Design review of the part built by this model. Coordinates are the model's own, in mm. Face numbers are marked on the shaded views. A direction names the side the tool comes from. Round coordinates to 2 decimals unless told otherwise and drop trailing zeros. Loops run counter-clockwise (first coordinate to the right, second up) from the corner with the lowest first, then second, coordinate; pieces in that order, holes last. Notation, with made-up numbers: (-10.5, 7) - (19.5, 7) arc R23 cw to (19.5, 17) - close; hole circle Ø5 at (40.25, 84). An arc over 180 degrees is marked (long way). Return JSON: item names as keys, results as strings. Group by question number.
(1) For the marked faces 1 and 2, list the 3-axis set-ups (+Z, -Z, +X, -X, +Y, -Y) from which the entire face can be reached by the end or side of a thin tool; tool diameter is ignored.
(2) We need section A-A, the plane x = 0. Write out the cut boundary in (y, z), and give its area (3 significant figures).
(3) We need section C-C, the plane y = 74. Write out the cut boundary in (x, z), and give its area (3 significant figures).
(4) Wall thickness on L1, parallel to Y at x = 8.35, z = 0; L2, parallel to X at y = 33.5, z = 0; L3, parallel to Z at x = -0.5, y = 9: over which ranges is each line inside the solid? List them lowest first. Write a range as [from, to].
(5) We need section B-B, the plane y = 62. Write out the cut boundary in (x, z), and give its area (3 significant figures).
(6) The part is to be moulded in two halves that separate along X. For the marked faces 3, 4 and 5, say which applies: pulls with the +X half, pulls with the -X half, needs draft (parallel to the pull), parting line crosses it, or undercut.
(7) Clearance check with flat-ended pins moving along their axes: pin 1 (1.5 mm diameter, centred on x = -5, y = 48.5, fed in from -Z); pin 2 (3 mm diameter, centred on y = 74, z = 0, fed in from +X); pin 3 (0.8 mm diameter, centred on y = -2, z = 0, fed in from +X); pin 4 (8 mm diameter, centred on y = 46.5, z = 6.5, fed in from +X). State where each tip first meets the part, or that it passes through.
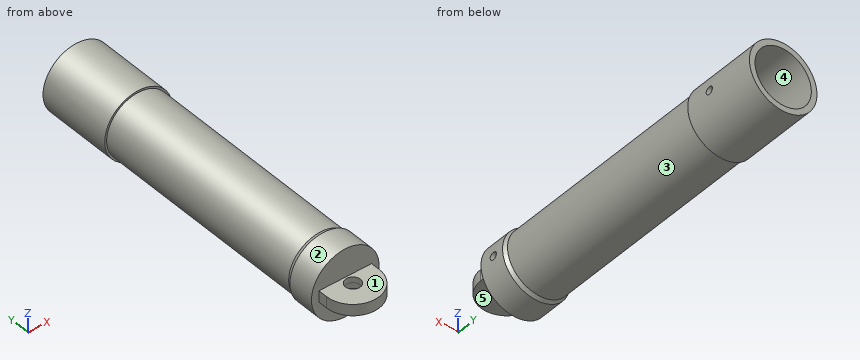
from build123d import *

# Parameters (mm, degrees)
SKETCH2_R                = 2
BOSS_EXTRUDE1_DEPTH      = 1.5
BOSS_EXTRUDE1_DEPTH_BACK = 1.5
SKETCH3_R                = 1
CUT_EXTRUDE1_DEPTH       = 50


with BuildPart() as part:
    # Sketch1 → Revolve1 (revolve)
    with BuildSketch(Plane.XY):
        Polygon((0, 0), (-9, 0), (-9, 7), (-8.5, 8), (-8.5, 67), (-9, 67), (-9, 87), (-7.5, 87), (-7.5, 2), (0, 2), align=None)
    revolve(axis=Axis((0, 87, 0), (0, -1, 0)))

    # Sketch2 → Boss-Extrude1 (add, two sides)
    with BuildSketch(Plane.XY) as boss_extrude1_sk:
        with BuildLine():
            Line((-7, 0), (7, 0))
            Line((7, 0), (7, -2.5))
            ThreePointArc((7, -2.5), (0, -9.5), (-7, -2.5))
            Line((-7, -2.5), (-7, 0))
        make_face()
        with Locations((0, -2.5)):
            Circle(SKETCH2_R, mode=Mode.SUBTRACT)
    extrude(amount=BOSS_EXTRUDE1_DEPTH)
    extrude(boss_extrude1_sk.sketch, amount=-BOSS_EXTRUDE1_DEPTH_BACK)

    # Sketch3 → Cut-Extrude1 (cut)
    with BuildSketch(Plane(origin=(0, 0, 0), x_dir=(0, 0, -1), z_dir=(1, 0, 0))):
        with Locations((0, 74)):
            Circle(SKETCH3_R)
        with Locations((0, 4)):
            Circle(SKETCH3_R)
    extrude(amount=CUT_EXTRUDE1_DEPTH, mode=Mode.SUBTRACT)


solid = part.part
Solutions:
{
 "1": {"face 1": "+Z, +X, -X, -Y", "face 2": "+Y, -Y"},
 "2": {"outline": "(-9.5, -1.5) - (-4.5, -1.5) - (-4.5, 1.5) - (-9.5, 1.5) - close; (-0.5, -1.5) - (0, -1.5) - (0, -9) - (7, -9) - (8, -8.5) - (67, -8.5) - (67, -9) - (87, -9) - (87, -7.5) - (2, -7.5) - (2, 7.5) - (87, 7.5) - (87, 9) - (67, 9) - (67, 8.5) - (8, 8.5) - (7, 9) - (0, 9) - (0, 1.5) - (-0.5, 1.5) - close", "area": "248 mm^2"},
 "3": {"outline": "(7.43, -1) arc R7.5 cw (long way) to (7.43, 1) - (8.94, 1) arc R9 ccw (long way) to (8.94, -1) - close", "area": "74.7 mm^2"},
 "4": {"L1": "[0, 3], [5, 73], [75, 87]", "L2": "[-8.5, -7.5], [7.5, 8.5]", "L3": "[-8.49, -7.48], [7.48, 8.49]"},
 "5": {"outline": "circle Ø17 at (0, 0); hole circle Ø15 at (0, 0)", "area": "50.3 mm^2"},
 "6": {"face 3": "parting line crosses it", "face 4": "undercut", "face 5": "needs draft"},
 "7": {"pin 1": "z = -7.36", "pin 2": "x = 9", "pin 3": "x = 7", "pin 4": "x = 8.12"}
}
